Source: CAD feature listing. Evaluate the final solid. Frame: model axes, mm. Coordinates: 2 decimals unless noted, no trailing zeros. Write each loop counter-clockwise with the first axis right and the second up, starting at its lowest first coordinate (ties: lowest second). Pieces come first, ordered by that corner, then holes. Notation, with made-up numbers: (28.25, 16.25) -> (61.25, 16.25) arc R24 cw to (61.25, 51.25) -> close; hole circle Ø6 at (19, 78). An arc over 180 degrees is marked (long way). One line per item, written item: value. Start each with the question number.
1. Line query: line 1 (Z direction, x = -20, y = 0.8); line 2 (Y direction, x = -6, z = -8.5); line 3 (Z direction, x = -20, y = 0.7). Output: solid intervals per line, ascending.
2. Section query D-D, the plane x = -14. Output: boundary loops of the cut face in (y, z).
3. Section query B-B, the plane x = -30. Output: boundary loops of the cut face in (y, z).
4. Mould query, pull axis X, two halves, no side actions, for faces 1 (the flat face through (-19, 0, -15)), 2 (the cylindrical face through (-34, 0.49, -8.02)), 3 (the flat face through (0, 0.7, -2.9)). Classes: released by +X, released by -X, zero draft, split by the parting line, or undercut.
5. Section query C-C, the plane y = -1.5. Output: boundary loops of the cut face in (x, z) (3 decimals), and give its area (3 significant figures).
6. First-contact query: P1, Ø4, axis at x = -20, y = -10, coming from the +Z side; P2, Ø8, axis at y = -9, z = -21, coming from the -X side; P3, Ø4, axis at x = -11.5, y = -7, coming from the +Z side. Flat tips, straight axial feed; report the tip coordinate or a pass-through.
7. Section query A-A, the plane z = -10.5. Output: boundary loops of the cut face in (x, y), and give its area (3 significant figures).
from build123d import *

# Parameters (mm, degrees)
SKETCH1_W           = 40
SKETCH1_H           = 40
SKETCH1_R           = 19
BOSS_EXTRUDE1_DEPTH = 1
BOSS_EXTRUDE3_DEPTH = 40
CUT_EXTRUDE1_DEPTH  = 40
SKETCH4_W           = 2
SKETCH4_H           = 17.959199538
CUT_EXTRUDE2_DEPTH  = 40
SKETCH5_W           = 4.291289536
SKETCH5_H           = 2.060082618
BOSS_EXTRUDE4_DEPTH = 1


with BuildPart() as part:
    # Sketch1 → Boss-Extrude1 (new body)
    with BuildSketch(Plane(origin=(0, 0, 0), x_dir=(1, 0, 0), z_dir=(0, 1, 0))):
        with Locations((-20, -4.822405003)):
            Rectangle(SKETCH1_W, SKETCH1_H)
        with Locations((-20, -4.822405003)):
            Circle(SKETCH1_R, mode=Mode.SUBTRACT)
    extrude(amount=BOSS_EXTRUDE1_DEPTH)

    # Sketch2 → Boss-Extrude3 (add)
    with BuildSketch(Plane(origin=(0, 0, 0), x_dir=(0, 0, -1), z_dir=(1, 0, 0))):
        Polygon((15.177594997, 0), (26.251567878, -16.654342515), (27.084285004, -16.100643871), (15.713552938, 1), (15.177594997, 1), align=None)
    extrude(amount=-BOSS_EXTRUDE3_DEPTH)

    # Sketch3 → Cut-Extrude1 (cut)
    with BuildSketch(Plane(origin=(0, 6.997999648, -10.524414707), x_dir=(1, 0, 0), z_dir=(0, -0.553698644, 0.832717126))):
        Polygon((-20, -28.40381377), (-40, -8.40381377), (-40, -28.40381377), align=None)
    extrude(amount=-CUT_EXTRUDE1_DEPTH, mode=Mode.SUBTRACT)

    # Sketch4 → Cut-Extrude2 (cut)
    with BuildSketch(Plane(origin=(0, 6.997999648, -10.524414707), x_dir=(1, 0, 0), z_dir=(0, -0.553698644, 0.832717126))):
        with Locations((-5, -18.291545123)):
            Rectangle(SKETCH4_W, SKETCH4_H)
    extrude(amount=-CUT_EXTRUDE2_DEPTH, mode=Mode.SUBTRACT)

    # Sketch5 → Boss-Extrude4 (add)
    with BuildSketch(Plane(origin=(0, 6.997999648, -10.524414707), x_dir=(1, 0, 0), z_dir=(0, -0.553698644, 0.832717126))):
        with Locations((-5.191272024, -19.192802864)):
            Rectangle(SKETCH5_W, SKETCH5_H)
    extrude(amount=-BOSS_EXTRUDE4_DEPTH)


solid = part.part
Computed values:
1. line 1: z = -15.85 to -14.18, 23.82 to 24.82
1. line 2: y = 0 to 1
1. line 3: z = -15.91 to -14.18, 23.82 to 24.82
2. outline: (-16.65, -26.25) -> (-16.1, -27.08) -> (1, -15.71) -> (1, -13.21) -> (0, -13.21) -> (0, -15.18) -> close; (0, 22.85) -> (1, 22.85) -> (1, 24.82) -> (0, 24.82) -> close
3. outline: (-8.33, -20.71) -> (-7.77, -21.55) -> (1, -15.71) -> (1, -11.33) -> (0, -11.33) -> (0, -15.18) -> close; (0, 20.98) -> (1, 20.98) -> (1, 24.82) -> (0, 24.82) -> close
4. face 1: zero draft
4. face 2: undercut
4. face 3: released by +X
5. outline: (-38.199, -16.175) -> (-37.534, -17.376) -> (-6, -17.376) -> (-6, -16.175) -> close; (-4, -17.376) -> (0, -17.376) -> (0, -16.175) -> (-4, -16.175) -> close
5. area: 43.1 mm²
6. P1: stops at z = -20.5
6. P2: stops at x = -33.28
6. P3: stops at z = -18.5
7. outline: (-40, 0) -> (-31.23, 0) -> (-31.23, 1) -> (-40, 1) -> close; (-8.77, 0) -> (0, 0) -> (0, 1) -> (-8.77, 1) -> close
7. area: 17.5 mm²
